from build123d import *

# Parameters (mm, degrees)
SKETCH1_W                    = 90
SKETCH1_H                    = 25
BOSS_EXTRUDE1_DEPTH          = 16.87
CUT_EXTRUDE2_DEPTH           = 4.5
ENL_V_MAT_EXTRU_1_DEPTH      = 34
FILLET1_RADIUS               = 12.5
FILLET1_LENGTH               = 11.75
ESQUISSE5_R                  = 1.75
ENL_V_MAT_EXTRU_4_DEPTH      = 50.65729453
FILLET3_R                    = 4
SKETCH8_W                    = 38.029495875
SKETCH8_H                    = 20.943583685
CUT_EXTRUDE6_DEPTH           = 2
ESQUISSE17_R                 = 6.45
ENL_V_MAT_EXTRU_7_DEPTH      = 3.6
ENL_V_MAT_EXTRU_8_DEPTH      = 50.65729453
ENL_V_MAT_EXTRU_8_DEPTH_BACK = 50.65729453
ESQUISSE18_R                 = 50
FILLET4_R                    = 0.5


with BuildPart() as part:
    # Sketch1 → Boss-Extrude1 (new body)
    with BuildSketch(Plane(origin=(0, 0, 0), x_dir=(1, 0, 0), z_dir=(0, 1, 0))):
        Rectangle(SKETCH1_W, SKETCH1_H)
    extrude(amount=BOSS_EXTRUDE1_DEPTH)

    # Sketch3 → Cut-Extrude2 (cut)
    with BuildSketch(Plane(origin=(0, 16.87, 0), x_dir=(1, 0, 0), z_dir=(0, 1, 0))):
        with BuildLine():
            Line((-39.272085844, 4.798838748), (-36.060975614, 5.136336504))
            ThreePointArc((-36.060975614, 5.136336504), (-32.500000002, 6.25), (-28.93902439, 5.136336506))
            Line((-28.93902439, 5.136336506), (-15, 2.5))
            ThreePointArc((-15, 2.5), (-12.5, 0), (-15, -2.5))
            Line((-15, -2.5), (-28.93902439, -5.136336506))
            ThreePointArc((-28.93902439, -5.136336506), (-32.500000002, -6.25), (-36.060975614, -5.136336504))
            Line((-36.060975614, -5.136336504), (-39.272085844, -4.798838748))
            ThreePointArc((-39.272085844, -4.798838748), (-40.8, 0), (-39.272085844, 4.798838748))
        make_face()
    extrude(amount=-CUT_EXTRUDE2_DEPTH, mode=Mode.SUBTRACT)

    # Esquisse2 → Enlèv. mat.-Extru.1 (cut)
    with BuildSketch(Plane.XY.offset(12.5)):
        Polygon((45, 16.87), (10, 16.87), (19, 7.87), (45, 7.87), align=None)
        Polygon((-45, 0), (10, 0), (4.88, 5.12), (-45, 5.12), align=None)
    extrude(amount=-ENL_V_MAT_EXTRU_1_DEPTH, mode=Mode.SUBTRACT)

    # Fillet1: full round fillet: the end face becomes a half cylinder, R = half its width
    fillet1_face = Plane((-45, 10.995, 0), x_dir=(0, -1, 0), z_dir=(-1, 0, 0))  # on the end face: x along it, z out of the body
    fillet1_slab = fillet1_face.offset(-FILLET1_RADIUS / 2) * Box(FILLET1_LENGTH, 2 * FILLET1_RADIUS, FILLET1_RADIUS, mode=Mode.PRIVATE)  # the body's end, R deep
    fillet1_round = Plane((-32.5, 10.995, 0), x_dir=(-1, 0, 0), z_dir=(0, -1, 0)) * Cylinder(FILLET1_RADIUS, FILLET1_LENGTH, mode=Mode.PRIVATE)  # its axis R under the face
    add(fillet1_slab - fillet1_round, mode=Mode.SUBTRACT)

    # Esquisse5 → Enlèv. mat.-Extru.4 (cut, through all)
    with BuildSketch(Plane(origin=(0, 0, 0), x_dir=(-1, 0, 0), z_dir=(0, -1, 0))):
        with Locations(Location((-40, 0, 0), (0, 0, 90))):
            Circle(ESQUISSE5_R)
    extrude(amount=-ENL_V_MAT_EXTRU_4_DEPTH, mode=Mode.SUBTRACT)

    # Fillet3
    fillet3_edges = [part.edges().sort_by_distance(p)[0] for p in [
        (45, 3.935, -12.5),
        (45, 3.935, 12.5),
    ]]
    fillet(fillet3_edges, radius=FILLET3_R)

    # Sketch8 → Cut-Extrude6 (cut)
    with BuildSketch(Plane(origin=(0, 16.87, 0), x_dir=(1, 0, 0), z_dir=(0, 1, 0))):
        with Locations((-5.673362901, 3.675760168)):
            Rectangle(SKETCH8_W, SKETCH8_H)
    extrude(amount=-CUT_EXTRUDE6_DEPTH, mode=Mode.SUBTRACT)

    # Esquisse17 → Enlèv. mat.-Extru.7 (cut)
    with BuildSketch(Plane.XZ.offset(-5.12)):
        with Locations((-32.5, 0)):
            Circle(ESQUISSE17_R)
    extrude(amount=-ENL_V_MAT_EXTRU_7_DEPTH, mode=Mode.SUBTRACT)

    # Esquisse18 → Enlèv. mat.-Extru.8 (cut, two sides: drawn at the far end of the back side and taken through both)
    with BuildSketch(Plane(origin=(0, 0, 0), x_dir=(1, 0, 0), z_dir=(0, 1, 0)).offset(-ENL_V_MAT_EXTRU_8_DEPTH_BACK)):
        with Locations((0, -50)):
            Circle(ESQUISSE18_R)
    extrude(amount=ENL_V_MAT_EXTRU_8_DEPTH + ENL_V_MAT_EXTRU_8_DEPTH_BACK, mode=Mode.SUBTRACT)

    # Fillet4
    fillet4_edges = [part.edges().sort_by_distance(p)[0] for p in [
        (-28.594055419, 16.87, -12.5),
        (19, 7.87, -4.37466216),
        (12, 14.87, -5.519322199),
        (-37.666530729, 16.87, -4.967587626),
        (-26.813567614, 16.87, -4.734341422),
        (-32.500000002, 16.87, -6.25),
        (-37.666530729, 16.87, 4.967587626),
        (-24.688110839, 16.87, 5.426249162),
        (-26.813567614, 16.87, 4.734341422),
        (-32.500000002, 16.87, 6.25),
        (-40.8, 16.87, 0),
        (-24.688110839, 16.87, -8.416173168),
        (-29.026696429, 16.87, 9.288197111),
        (-44.996887004, 16.87, -0.278953754),
    ]]
    fillet(fillet4_edges, radius=FILLET4_R)


solid = part.part
Source: CAD feature listing. Evaluate the final solid. Frame: model axes, mm. A direction names the side the tool comes from. Give positions to 0.01 mm unless a question says otherwise; leave off trailing zeros. Write each loop counter-clockwise with the first axis right and the second up, starting at its lowest first coordinate (ties: lowest second). Pieces come first, ordered by that corner, then holes. Notation, with made-up numbers: (64, -2) -> (117, -2) arc R17 ccw to (117, 21) -> close; hole circle Ø7 at (-5.5, -2.75). An arc over 180 degrees is marked (long way). Return JSON: item names as keys, results as strings. Group by question number.
1. Section B-B, the plane y = 3. Output: boundary loops of the cut face in (x, z).
2. Section A-A, the plane x = 40. Output: boundary loops of the cut face in (y, z).
3. Pin query (flat end, axial travel): pin 1 Ø1.9 at (x, z) = (-21.5, 5.5) entering from +Y; pin 2 Ø6 at (x, z) = (-32.5, 2) entering from +Y; pin 3 Ø6.5 at (x, z) = (-34, -2) entering from -Y. Return the tip coordinate at first contact, or that it passes through.
4. Mould query, pull axis X, two halves, no side actions, for faces 1 (the face through (7, 3, -6)), 2 (the face through (15.45, 11.42, -4.29)), 3 (the face through (-37.689, 14.398, -4.965)). Classes: +X half, -X half, draft (parallel to the pull), parting line (faces both ways), or undercut.
5. Access query for faces 4 (the face through (32, 7.87, 0)), 5 (the face through (-22.067, 13.954, -3.837)), 6 (the face through (-26.35, 6.89, 1.94)). Directions: +Z, -Z, +X, -X, +Y, -Y. A direction counts if a zero-diameter tool reaches every point of the face in a straight line with its end or side. Return the directions, or none.
6. Material intervals for line 1 (Y direction, x = -21.5, z = 2.25); line 2 (Z direction, x = -28.5, y = 7); line 3 (X direction, y = 7.25, z = -3), sorted ascending. Write a range as from..to.
Determined:
{
 "1": {"outline": "(7, -12.5) -> (41, -12.5) arc R4 ccw to (45, -8.5) -> (45, 8.5) arc R4 ccw to (41, 12.5) -> (33.07, 12.5) arc R50 cw to (7, 0.49) -> close; hole circle Ø3.5 at (40, 0)"},
 "2": {"outline": "(0, -12.5) -> (7.87, -12.5) -> (7.87, -1.75) -> (0, -1.75) -> close; (0, 1.75) -> (7.87, 1.75) -> (7.87, 12.5) -> (0, 12.5) -> close"},
 "3": {"pin 1": "stops at y = 14.87", "pin 2": "stops at y = 12.37", "pin 3": "stops at y = 8.72"},
 "4": {"face 1": "-X half", "face 2": "+X half", "face 3": "undercut"},
 "5": {"face 4": "+Z, -Z, +X, +Y", "face 5": "+Y", "face 6": "-Y"},
 "6": {"line 1": "y = 5.12..12.37", "line 2": "z = -12.5..-5.06, 5.06..8.92", "line 3": "x = -44.63..-38.21, -26.79..45"}
}
